from build123d import *

# Parameters (mm, degrees)
SKETCH_9_R               = 72
SKETCH_9_R_2             = 70
EXTRUDE_9_DEPTH          = 10
SKETCH_9_18_R            = 70
SKETCH_9_18_R_2          = 66
EXTRUDE_10_DEPTH         = 2.5
SKETCH_9_19_R            = 66
EXTRUDE_11_DEPTH         = 10
SHELL_START              = -10
SHELL_2_OUTLINE_R        = 64
SHELL_2_DEPTH            = 8
F_2_5MM_1_REACH          = 163.118
F_2_5MM_1_BORE_R         = 1.25
PATTERN_CIRCULAR_1_COUNT = 4
SKETCH_15_W              = 1
SKETCH_15_H              = 2


# Read off the part's stored shape, not the designer's step: 薄殼2
with BuildPart() as part:
    # 草圖9 → 填料-伸長9 (new body)
    with BuildSketch(Plane(origin=(0, 0, 0), x_dir=(1, 0, 0), z_dir=(0, 1, 0))):
        with Locations(Location((0, 0, 0), (0, 0, 270))):
            Circle(SKETCH_9_R)
        with Locations(Location((0, 0, 0), (0, 0, 270))):
            Circle(SKETCH_9_R_2, mode=Mode.SUBTRACT)
    extrude(amount=-EXTRUDE_9_DEPTH)

    # 草圖9<18> → 填料-伸長10 (add)
    with BuildSketch(Plane(origin=(0, 0, 0), x_dir=(1, 0, 0), z_dir=(0, 1, 0))):
        with Locations(Location((0, 0, 0), (0, 0, 270))):
            Circle(SKETCH_9_18_R)
        with Locations(Location((0, 0, 0), (0, 0, 270))):
            Circle(SKETCH_9_18_R_2, mode=Mode.SUBTRACT)
    extrude(amount=-EXTRUDE_10_DEPTH)

    # 草圖9<19> → 填料-伸長11 (add)
    with BuildSketch(Plane(origin=(0, 0, 0), x_dir=(1, 0, 0), z_dir=(0, 1, 0))):
        with Locations(Location((0, 0, 0), (0, 0, 270))):
            Circle(SKETCH_9_19_R)
    extrude(amount=-EXTRUDE_11_DEPTH)

    # 薄殼2 outline → 薄殼2 (cut)
    with BuildSketch(Plane(origin=(0, 0, 0), x_dir=(1, 0, 0), z_dir=(0, 1, 0)).offset(SHELL_START)):
        Circle(SHELL_2_OUTLINE_R)
    extrude(amount=SHELL_2_DEPTH, mode=Mode.SUBTRACT)

    # Ø2.5mm 定位孔1 bore (on position points) → Ø2.5mm 定位孔1 (cut, up to next)
    with BuildSketch(Plane(origin=(0, -6.25, 72), x_dir=(1, 0, 0), z_dir=(0, 0, 1)), mode=Mode.PRIVATE) as f_2_5mm_1_sk1:
        Circle(F_2_5MM_1_BORE_R)
    f_2_5mm_1_tool1 = extrude(f_2_5mm_1_sk1.sketch, amount=-F_2_5MM_1_REACH, mode=Mode.PRIVATE) & part.part
    f_2_5mm_1 = f_2_5mm_1_tool1.solids().sort_by_distance((0, -6.25, 72))[0]
    add(f_2_5mm_1, mode=Mode.SUBTRACT)

    # 環狀複製排列1: Ø2.5mm 定位孔1 ×4 about axis
    pattern_circular_1_axis = Axis((0, -10, 0), (0, 1, 0))
    for i in range(1, PATTERN_CIRCULAR_1_COUNT):
        add(f_2_5mm_1.rotate(pattern_circular_1_axis, i * 360 / PATTERN_CIRCULAR_1_COUNT), mode=Mode.SUBTRACT)

    # 草圖15 → 除料-旋轉2 (revolve, cut)
    with BuildSketch(Plane(origin=(0, 0, 0), x_dir=(0, 0, -1), z_dir=(1, 0, 0))):
        with Locations((-71.5, -2)):
            Rectangle(SKETCH_15_W, SKETCH_15_H)
    revolve(axis=Axis((0, 0, 0), (0, -1, 0)), mode=Mode.SUBTRACT)


solid = part.part
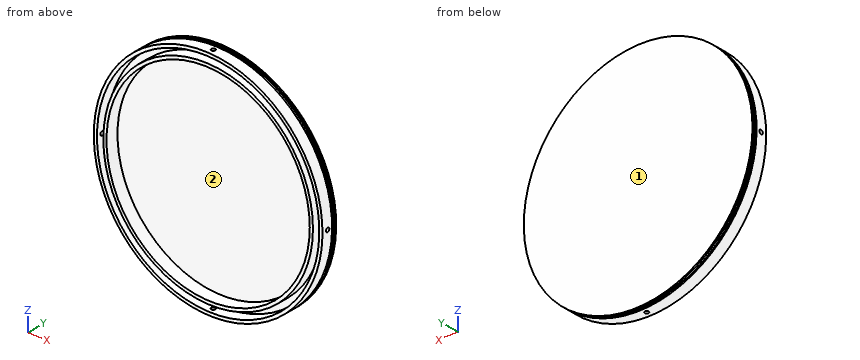
Could you check a few things on this model? Use its own coordinates, in mm. Face numbers are marked on the shaded views. Give positions to 0.01 mm unless a question says otherwise; leave off trailing zeros. Order: outer loops, then holes, each group sorted by start corner. A loop starts at its lowest first (then second) coordinate and runs counter-clockwise, first axis right, second up.
1. Suppose I cut it at A-A (z = -37). List the corners of the cut face in (x, y) for me, plus the area to 3 significant figures.
2. I need wall thicknesses on L1, parallel to X at y = -3.5, z = 0; L2, parallel to X at y = -8.25, z = 22; L3, parallel to Y at x = 0, z = 70.8. Which ranges of each line are inside material? Lowest first, please.
3. We'd pull the mould along Z, two halves only. Please class the marked faces 1 and 2: pulls with the +Z half, pulls with the -Z half, needs draft (parallel to the pull), parting line crosses it, or undercut.
4. Will these pins go through, and if not, where does the flat tip stop? P1, Ø1.5, axis at x = -41.5, y = -7, coming from the +Z side; P2, Ø6, axis at x = -6.5, z = -8.5, coming from the +Y side; P3, Ø6, axis at y = -2, z = 55, coming from the -X side; P4, Ø2, axis at x = 0, y = -6.25, coming from the +Z side.
5. Suppose I cut it at B-B (x = 4.5). List the corners of the cut face in (y, z) for me, plus the area to 3 significant figures.
Solved:
1. outline: (-61.77, -10) - (-59.42, -10) - (-59.42, -2.5) - (-54.65, -2.5) - (-54.65, -10) - (-52.22, -10) - (-52.22, -2) - (52.22, -2) - (52.22, -10) - (54.65, -10) - (54.65, -2.5) - (59.42, -2.5) - (59.42, -10) - (61.77, -10) - (61.77, -3) - (60.6, -3) - (60.6, -1) - (61.77, -1) - (61.77, 0) - (-61.77, 0) - (-61.77, -1) - (-60.6, -1) - (-60.6, -3) - (-61.77, -3) - close
1. area: 324 mm2
2. L1: x = -72 to -70, -66 to -64, 64 to 66, 70 to 72
2. L2: x = -68.56 to -66.45, -62.23 to -60.1, 60.1 to 62.23, 66.45 to 68.56
2. L3: y = -10 to -7.5, -5 to 0
3. face 1: needs draft
3. face 2: undercut
4. P1: stops at z = 59.36
4. P2: stops at y = 0
4. P3: stops at x = -49.62
4. P4: stops at z = 66
5. outline: (-10, -71.86) - (-3, -71.86) - (-3, -70.86) - (-1, -70.86) - (-1, -71.86) - (0, -71.86) - (0, 71.86) - (-1, 71.86) - (-1, 70.86) - (-3, 70.86) - (-3, 71.86) - (-10, 71.86) - (-10, 69.86) - (-2.5, 69.86) - (-2.5, 65.85) - (-10, 65.85) - (-10, 63.84) - (-2, 63.84) - (-2, -63.84) - (-10, -63.84) - (-10, -65.85) - (-2.5, -65.85) - (-2.5, -69.86) - (-10, -69.86) - close
5. area: 352 mm2
